Autodesk Inventor part; units mm, degrees
ref_plane "YZ Plane" through (0, 0, 0) normal (1, 0, 0) x (0, 1, 0)
ref_plane "XZ Plane" through (0, 0, 0) normal (0, 1, 0) x (-1, 0, 0)
ref_plane "XY Plane" through (0, 0, 0) normal (0, 0, 1) x (1, 0, 0)
sketch "Sketch1" plane through (0, 0, 0) normal (0, 1, 0) x (-1, 0, 0)
  line L0 (44, 0) -> (44, -20)
  line L1 (44, -20) -> (47, -20)
  line L2 (47, -20) -> (47, -30)
  line L3 (47, -30) -> (44, -30)
  line L4 (44, -30) -> (44, -50)
  line L5 (44, -50) -> (27, -50)
  line L6 (27, -50) -> (27, -47)
  line L7 (27, -47) -> (17, -47)
  line L8 (17, -47) -> (17, -50)
  line L9 (17, -50) -> (0, -50)
  line L10 (0, -50) -> (0, -30)
  line L11 (0, -30) -> (-3, -30)
  line L12 (-3, -30) -> (-3, -20)
  line L13 (-3, -20) -> (0, -20)
  line L14 (0, -20) -> (0, 0)
  line L15 (44, 0) -> (27, 0)
  line L16 (27, 0) -> (27, -3)
  line L17 (27, -3) -> (17, -3)
  line L18 (17, -3) -> (17, 0)
  line L19 (17, 0) -> (0, 0)
  line L20 (27, -42.5) -> (17, -42.5)
  line L21 (17, -42.5) -> (17, -37.5)
  line L22 (17, -37.5) -> (27, -37.5)
  line L23 (27, -37.5) -> (27, -42.5)
  point P0 (47, -25)
  point P1 (22, -3)
  point P2 (22, -47)
  point P3 (22, -42.5)
  dimension "d0" = 3
  dimension "d1" = 10
  dimension "d2" = 3
  dimension "d3" = 50
  dimension "d4" = 10
  dimension "d5" = 50
  dimension "d7" = 10
  dimension "d8" = 5
  dimension "d9" = 4.5
extrude "Extrusion1" add sketch "Sketch1" along normal blind 3
Source: CAD feature listing. Evaluate the final solid. Frame: model axes, mm. A direction names the side the tool comes from. Give positions to 0.01 mm unless a question says otherwise; leave off trailing zeros. Loops run counter-clockwise (first coordinate to the right, second up) from the corner with the lowest first, then second, coordinate; pieces in that order, holes last. Notation, with made-up numbers: (25.25, -33.75) -> (53.25, -33.75) arc R14 ccw to (53.25, -25.75) -> close; hole circle Ø10 at (3, 6.25). An arc over 180 degrees is marked (long way). Use a Markdown table: item, result. Add a question column.
(1) Section query D-D (z = -14). Output: boundary loops of the cut face in (x, y).
(2) Section query C-C (y = 1.25). Output: boundary loops of the cut face in (x, z), then the cut area to 3 significant figures.
(3) Section query B-B (z = -40). Output: boundary loops of the cut face in (x, y).
(4) Ray query, line 1 (X direction, y = 1.2, z = -38); line 2 (X direction, y = 0.8, z = -34); line 3 (Z direction, x = -20.5, y = 0.1). Return the intervals inside material, ascending.
(5) Section query A-A (x = -24.5). Output: boundary loops of the cut face in (y, z).
(6) First-contact query: pin 1 Ø0.9 at (y, z) = (1.5, -39) entering from +X; pin 2 Ø0.9 at (y, z) = (1, -1) entering from -X. Flat tips, straight axial feed; report the tip coordinate or a pass-through.
(7) Access query for faces 1 (the face through (-22, 1, -47)), 2 (the face through (0, 1, -10)), 3 (the face through (-44, 1, -40)), 4 (the face through (0, 1, -40)). Directions: +Z, -Z, +X, -X, +Y, -Y. A direction counts if a zero-diameter tool reaches every point of the face in a straight line with its end or side. Return the directions, or none.
Checked values:
| question | item | result |
|---|---|---|
| 1 | outline | (-44, 0) -> (0, 0) -> (0, 3) -> (-44, 3) -> close |
| 2 | outline | (-47, -30) -> (-44, -30) -> (-44, -50) -> (-27, -50) -> (-27, -47) -> (-17, -47) -> (-17, -50) -> (0, -50) -> (0, -30) -> (3, -30) -> (3, -20) -> (0, -20) -> (0, 0) -> (-17, 0) -> (-17, -3) -> (-27, -3) -> (-27, 0) -> (-44, 0) -> (-44, -20) -> (-47, -20) -> close; hole (-27, -42.5) -> (-17, -42.5) -> (-17, -37.5) -> (-27, -37.5) -> close |
| 2 | area | 2,150 mm^2 |
| 3 | outline | (-44, 0) -> (-27, 0) -> (-27, 3) -> (-44, 3) -> close; (-17, 0) -> (0, 0) -> (0, 3) -> (-17, 3) -> close |
| 4 | line 1 | -44 to -27, -17 to 0 |
| 4 | line 2 | -44 to 0 |
| 4 | line 3 | -47 to -42.5, -37.5 to -3 |
| 5 | outline | (0, -47) -> (3, -47) -> (3, -42.5) -> (0, -42.5) -> close; (0, -37.5) -> (3, -37.5) -> (3, -3) -> (0, -3) -> close |
| 6 | pin 1 | x = 0 |
| 6 | pin 2 | x = -44 |
| 7 | face 1 | -Z, +Y, -Y |
| 7 | face 2 | +Z, +X, +Y, -Y |
| 7 | face 3 | -Z, -X, +Y, -Y |
| 7 | face 4 | -Z, +X, +Y, -Y |
